Geometry: final body of the model. Coordinates: model frame, mm. A direction names the side the tool comes from. Give positions to 0.01 mm unless a question says otherwise; leave off trailing zeros. Write each loop counter-clockwise with the first axis right and the second up, starting at its lowest first coordinate (ties: lowest second). Pieces come first, ordered by that corner, then holes.
```python
from build123d import *

# Parameters (mm, degrees)
F1_DEPTH = 950
F2_W     = 988
F2_H     = 10
F3_DEPTH = 15
F4_SIZE  = 5


with BuildPart() as f1:
    # F0 (on Right) → F1 (new body)
    with BuildSketch(Plane.YZ):
        with BuildLine():
            ThreePointArc((0, -1), (-0.292893, -0.292893), (-1, 0))
            Line((-1, 0), (-30, 0))
            Line((-30, 0), (-46, -2.821232))
            Line((-46, -2.821232), (-46, -5.181976))
            Line((-46, -5.181976), (-15, -13.5))
            Line((-15, -13.5), (-15, -45))
            Line((-15, -45), (0, -45))
            Line((0, -45), (0, -1))
        make_face()
    extrude(amount=-F1_DEPTH)

    # F2 (on Front) → F3 (join)
    with BuildSketch(Plane.XZ):
        with Locations((-475, -40)):
            Rectangle(F2_W, F2_H)
    extrude(amount=F3_DEPTH)

    # F4
    f4_edges = [f1.edges().sort_by_distance(p)[0] for p in [
        (0, -46, -4.001604),
        (-950, -46, -4.001604),
    ]]
    chamfer(f4_edges, length=F4_SIZE)


solid = f1.part
```
Item 1: Section B-B, the plane z = -21. Return the cut outline in (x, y).
Found:
outline: (-950, -15) - (0, -15) - (0, 0) - (-950, 0) - close
Item 2: Pin query (flat end, axial travel): pin 1 Ø16.5 at (x, y) = (10.5, -11) entering from +Z; pin 2 Ø12 at (x, z) = (-741.5, -30) entering from -Y. Return the tip coordinate at first contact, or that it passes through.
Found:
pin 1: stops at z = -35
pin 2: stops at y = -15
Item 3: Section A-A, the plane x = -655.5. Return the cut outline in (y, z), plus the area to 3 significant figures.
Found:
outline: (-46, -5.18) - (-15, -13.5) - (-15, -45) - (0, -45) - (0, -1) arc R1 ccw to (-1, 0) - (-30, 0) - (-46, -2.82) - close
area: 942 mm2
Item 4: Reachability of faces 1 (the face through (-950, -12, -13)), 2 (the face through (9, -7, -35)), 3 (the face through (-482, -15, -29)), 4 (the face through (-468.35, -37.89, -1.39)) from +Z, -Z, +X, -X, +Y, -Y: full face, straight path, thin tool, end or side. Return the list, or none.
Found:
face 1: +Z, -X, +Y, -Y
face 2: +Z, +X, +Y, -Y
face 3: -Z, +X, -X, -Y
face 4: +Z, +X, -X, -Y
Item 5: Line query: L1, parallel to Y at x = -433, z = -26; L2, parallel to X at y = -24, z = -7; L3, parallel to Z at x = -587, y = -40.5. Output: solid intervals per line, ascending.
Found:
L1: y = -15 to 0
L2: x = -950 to 0
L3: z = -6.66 to -1.85
